The listing builds one solid part. Answer for the finished solid, in the listing's coordinates (mm). Face numbers are marked on the shaded views. A direction names the side the tool comes from. Coordinates: 2 decimals unless noted, no trailing zeros. Order: outer loops, then holes, each group sorted by start corner. A loop starts at its lowest first (then second) coordinate and runs counter-clockwise, first axis right, second up. Notation, with made-up numbers: (-30.5, 39) -> (-3.5, 39) arc R11 ccw to (-3.5, 57) -> close; hole circle Ø7 at (68, -27). An arc over 180 degrees is marked (long way). Return JSON: item names as keys, results as strings.
from build123d import *

# Parameters (mm, degrees)
F0_R     = 8
F1_DEPTH = 15
F0_W     = 45
F0_H     = 20
F0_R_2   = 1
F2_DEPTH = 1.2
F3_R     = 0.5


with BuildPart() as f1:
    # F0 (on Front) → F1 (new body)
    with BuildSketch(Plane.XZ):
        with Locations((-13.5, 0)):
            Circle(F0_R)
    extrude(amount=F1_DEPTH)



with BuildPart() as f1b:
    # F0 (on Front) → F1, piece 2 (new body)
    with BuildSketch(Plane.XZ):
        with Locations((13.5, 0)):
            Circle(F0_R)
    extrude(amount=F1_DEPTH)


with BuildPart() as f1_1:
    add(f1.part)

    add(f1b.part)  # F2 merges F1b
    # F0 (on Front) → F2 (join)
    with BuildSketch(Plane.XZ):
        Rectangle(F0_W, F0_H)
        with Locations((-20, -7.5)):
            Circle(F0_R_2, mode=Mode.SUBTRACT)
        with Locations((-13.5, 0)):
            Circle(F0_R, mode=Mode.SUBTRACT)
        with Locations((13.5, 0)):
            Circle(F0_R, mode=Mode.SUBTRACT)
        with Locations((20, 7.5)):
            Circle(F0_R_2, mode=Mode.SUBTRACT)
    extrude(amount=F2_DEPTH)

    # F3
    f3_edges = [f1_1.edges().sort_by_distance(p)[0] for p in [
        (-21.5, -15, 0),
        (5.5, -15, 0),
    ]]
    fillet(f3_edges, radius=F3_R)


solid = f1_1.part
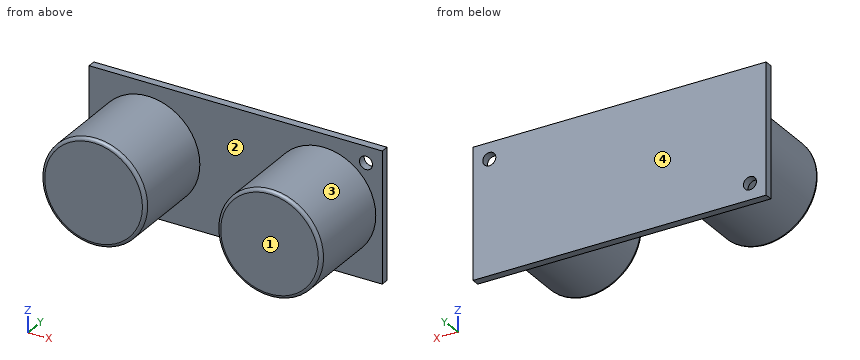
1. The part is cut by section B-B on z = 0. Give the vertices of the cut face in (x, y), and give its area (3 significant figures).
Answer block:
{"outline": "(-22.5, -1.2) -> (-21.5, -1.2) -> (-21.5, -14.5) arc R0.5 ccw to (-21, -15) -> (-6, -15) arc R0.5 ccw to (-5.5, -14.5) -> (-5.5, -1.2) -> (5.5, -1.2) -> (5.5, -14.5) arc R0.5 ccw to (6, -15) -> (21, -15) arc R0.5 ccw to (21.5, -14.5) -> (21.5, -1.2) -> (22.5, -1.2) -> (22.5, 0) -> (-22.5, 0) -> close", "area": "495 mm2"}
2. The part is cut by section C-C on y = -6.25. Give the vertices of the cut face in (x, z).
Answer block:
{"outline": "circle Ø16 at (-13.5, 0); circle Ø16 at (13.5, 0)"}
3. For the marked faces 3 and 4, determine the directions among +Z, -Z, +X, -X, +Y, -Y from which every point of the face is accessible in a straight line to the end or side of a thin tool.
Answer block:
{"face 3": "-Y", "face 4": "+Z, -Z, +X, -X, +Y"}
4. Determine the mould class of the marked faces 1 and 2 for opening direction X: pulls with the +X half, pulls with the -X half, needs draft (parallel to the pull), parting line crosses it, or undercut.
Answer block:
{"face 1": "needs draft", "face 2": "undercut"}
5. Each of these flat-tipped pins is pushed along its axis until it touches: pin 1 Ø5 at (y, z) = (-8.5, 1) entering from -X; pin 2 Ø6 at (x, z) = (-10, -0.5) entering from +Y; pin 3 Ø4 at (x, z) = (-0.5, -8) entering from -Y; pin 4 Ø1 at (x, y) = (-15, -6) entering from +Z. Where does it stop, or does it pass through?
Answer block:
{"pin 1": "stops at x = -21.5", "pin 2": "stops at y = 0", "pin 3": "stops at y = -1.2", "pin 4": "stops at z = 7.94"}
6. The part is cut by section D-D on x = -2. Give the vertices of the cut face in (y, z), and give its area (3 significant figures).
Answer block:
{"outline": "(-1.2, -10) -> (0, -10) -> (0, 10) -> (-1.2, 10) -> close", "area": "24.0 mm2"}
7. The part is cut by section A-A on x = -13.5. Give the vertices of the cut face in (y, z).
Answer block:
{"outline": "(-15, -7.5) arc R0.5 ccw to (-14.5, -8) -> (-1.2, -8) -> (-1.2, -10) -> (0, -10) -> (0, 10) -> (-1.2, 10) -> (-1.2, 8) -> (-14.5, 8) arc R0.5 ccw to (-15, 7.5) -> close"}
8. Consider line 1 (Z direction, x = -20, y = -0.5); line 2 (Z direction, x = 20, y = -0.3); line 3 (X direction, y = -12.5, z = 4). Determine where each line is inside the solid, lowest interval first. Write a range as from..to.
Answer block:
{"line 1": "z = -10..-8.5, -6.5..10", "line 2": "z = -10..6.5, 8.5..10", "line 3": "x = -20.43..-6.57, 6.57..20.43"}
